Work out the finished part from the listing and answer in its coordinate system (mm). Face numbers are marked on the shaded views. A direction names the side the tool comes from. Give positions to 0.01 mm unless a question says otherwise; leave off trailing zeros. Order: outer loops, then holes, each group sorted by start corner. A loop starts at its lowest first (then second) coordinate and runs counter-clockwise, first axis right, second up. Notation, with made-up numbers: (41.25, -33) - (99.25, -33) arc R19 ccw to (99.25, -7) - close; hole circle Ø8 at (36, 81.5). An arc over 180 degrees is marked (long way). Return JSON: item names as keys, results as strings. Group by question number.
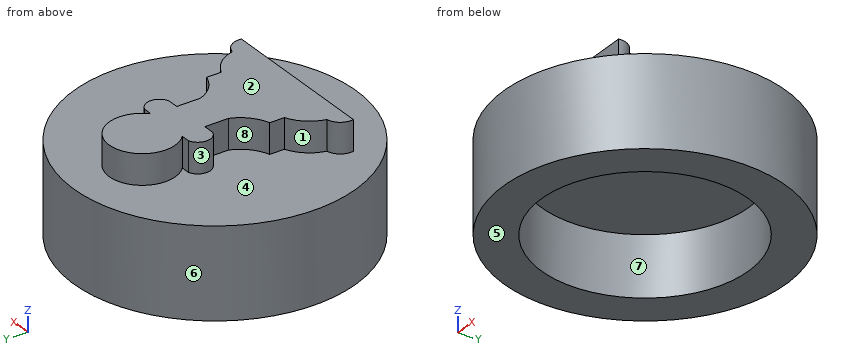
from build123d import *

# Parameters (mm, degrees)
SKETCH1_R           = 11.938
SKETCH1_R_2         = 8.763
BOSS_EXTRUDE1_DEPTH = 5.08
SKETCH2_R           = 11.938
BOSS_EXTRUDE2_DEPTH = 2.54
BOSS_EXTRUDE3_DEPTH = 2.54


with BuildPart() as part:
    # Sketch1 → Boss-Extrude1 (new body)
    with BuildSketch(Plane.XY):
        Circle(SKETCH1_R)
        Circle(SKETCH1_R_2, mode=Mode.SUBTRACT)
    extrude(amount=BOSS_EXTRUDE1_DEPTH)

    # Sketch2 → Boss-Extrude2 (add)
    with BuildSketch(Plane.XY.offset(5.08)):
        Circle(SKETCH2_R)
    extrude(amount=BOSS_EXTRUDE2_DEPTH)

    # Sketch3 → Boss-Extrude3 (add)
    with BuildSketch(Plane.XY.offset(7.62)):
        with BuildLine():
            Line((6.799209261, -6.976502995), (-6.799209261, -6.976502995))
            ThreePointArc((-6.799209261, -6.976502995), (-6.57773466, -5.997747251), (-5.729043644, -5.462268619))
            ThreePointArc((-5.729043644, -5.462268619), (-5.055714591, -4.101642026), (-3.830122247, -3.205762488))
            Line((-3.830122247, -3.205762488), (-3.830122247, -1.958745943))
            ThreePointArc((-3.830122247, -1.958745943), (-2.529170198, -1.211237743), (-1.703785584, 0.041752673))
            Line((-1.703785584, 0.041752673), (-1.703785584, 2.042251288))
            Line((-1.703785584, 2.042251288), (-2.652822308, 2.042251288))
            ThreePointArc((-2.652822308, 2.042251288), (-3.394876144, 3.066744886), (-2.652822308, 4.091238485))
            Line((-2.652822308, 4.091238485), (-1.910768473, 4.091238485))
            ThreePointArc((-1.910768473, 4.091238485), (0, 8.941901019), (1.910768473, 4.091238485))
            Line((1.910768473, 4.091238485), (2.652822308, 4.091238485))
            ThreePointArc((2.652822308, 4.091238485), (3.394876144, 3.066744886), (2.652822308, 2.042251288))
            Line((2.652822308, 2.042251288), (1.703785584, 2.042251288))
            Line((1.703785584, 2.042251288), (1.703785584, 0.041752673))
            ThreePointArc((1.703785584, 0.041752673), (2.529170198, -1.211237743), (3.830122247, -1.958745943))
            Line((3.830122247, -1.958745943), (3.830122247, -3.205762488))
            ThreePointArc((3.830122247, -3.205762488), (5.055714591, -4.101642026), (5.729043644, -5.462268619))
            ThreePointArc((5.729043644, -5.462268619), (6.57773466, -5.997747251), (6.799209261, -6.976502995))
        make_face()
    extrude(amount=BOSS_EXTRUDE3_DEPTH)


solid = part.part
1. Each of these flat-tipped pins is pushed along its axis until it touches: pin 1 (1 mm diameter, centred on x = -2, z = 8.5, fed in from -Y); pin 2 (1.6 mm diameter, centred on y = 1.5, z = 9.5, fed in from -X); pin 3 (3 mm diameter, centred on x = 2, z = 8, fed in from +Y). Where does it stop, or does it pass through?
2. The part is cut by section B-B (x = 0). Give the vertices of the cut face in (y, z).
3. The part is cut by section C-C (y = 3.25). Give the vertices of the cut face in (x, z), and give its area (3 significant figures).
4. Determine the mould class of the marked faces 1, 2 and 3 for opening direction Y: released by +Y, released by -Y, zero draft, split by the parting line, or undercut.
5. Consider probe 1 along Y at (x, z) = (2.25, 9.75); probe 2 along Y at (x, z) = (0, 3.3); probe 3 along Z at (x, y) = (-4.25, 3.5). Determine where each line is inside the solid, lowest interval first. Write a range as from..to.
6. The part is cut by section A-A (z = 9). Give the vertices of the cut face in (x, y), and give its area (3 significant figures).
7. The part is cut by section D-D (z = 1.75). Give the vertices of the cut face in (x, y), and give its area (3 significant figures).
8. A tool of negligible diameter and unlimited length cuts with its end or side. For the marked faces 4, 5, 6, 7 and 8, from which of +Z, -Z, +X, -X, +Y, -Y can it reach the whole face along a straight path? Write none if from no direction.
Answers:
{
 "1": {"pin 1": "stops at y = -6.98", "pin 2": "stops at x = -3.07", "pin 3": "stops at y = 11.93"},
 "2": {"outline": "(-11.94, 0) - (-8.76, 0) - (-8.76, 5.08) - (8.76, 5.08) - (8.76, 0) - (11.94, 0) - (11.94, 7.62) - (8.94, 7.62) - (8.94, 10.16) - (-6.98, 10.16) - (-6.98, 7.62) - (-11.94, 7.62) - close"},
 "3": {"outline": "(-11.49, 0) - (-8.14, 0) - (-8.14, 5.08) - (8.14, 5.08) - (8.14, 0) - (11.49, 0) - (11.49, 7.62) - (3.38, 7.62) - (3.38, 10.16) - (-3.38, 10.16) - (-3.38, 7.62) - (-11.49, 7.62) - close", "area": "110 mm^2"},
 "4": {"face 1": "released by +Y", "face 2": "zero draft", "face 3": "undercut"},
 "5": {"probe 1": "y = -6.98..-0.91, 2.04..4.09, 4.47..7.81", "probe 2": "y = -11.94..-8.76, 8.76..11.94", "probe 3": "z = 5.08..7.62"},
 "6": {"outline": "(-6.8, -6.98) - (6.8, -6.98) arc R1.31 ccw to (5.73, -5.46) arc R3.19 ccw to (3.83, -3.21) - (3.83, -1.96) arc R3.24 cw to (1.7, 0.04) - (1.7, 2.04) - (2.65, 2.04) arc R1.08 ccw to (2.65, 4.09) - (1.91, 4.09) arc R2.8 ccw (long way) to (-1.91, 4.09) - (-2.65, 4.09) arc R1.08 ccw to (-2.65, 2.04) - (-1.7, 2.04) - (-1.7, 0.04) arc R3.24 cw to (-3.83, -1.96) - (-3.83, -3.21) arc R3.19 ccw to (-5.73, -5.46) arc R1.31 ccw to start", "area": "105 mm^2"},
 "7": {"outline": "circle Ø23.88 at (0, 0); hole circle Ø17.53 at (0, 0)", "area": "206 mm^2"},
 "8": {"face 4": "+Z", "face 5": "-Z, +X, -X, +Y, -Y", "face 6": "+Z, -Z", "face 7": "-Z", "face 8": "+Z, -X"}
}
